CAD build for the part. Positions are in the model's coordinates, mm. A direction names the side the tool comes from. Round coordinates to 2 decimals unless told otherwise and drop trailing zeros. Order: outer loops, then holes, each group sorted by start corner. A loop starts at its lowest first (then second) coordinate and runs counter-clockwise, first axis right, second up. Notation, with made-up numbers: (-3, 66.25) -> (33, 66.25) arc R22 ccw to (33, 103.25) -> close; hole circle Ø4 at (-12.5, -4.75). An arc over 180 degrees is marked (long way). Return JSON: item names as keys, results as strings. Group by question number.
Q1. Flat gauge pins, fed straight in: pin 1 (1.2 mm diameter, centred on x = 84.5, z = 1.5, fed in from -Y); pin 2 (5 mm diameter, centred on x = 53.5, y = 19.25, fed in from +Z); pin 3 (2.5 mm diameter, centred on x = 4.5, y = 19.25, fed in from -Z). Where does each tip first touch, or does it go through?
Q2. Which spindle directions (+Z, -Z, +X, -X, +Y, -Y) get a long thin tool onto all of the face, cutting with end or side? Do faces 1 (the flat face through (29, 0, 2)), 2 (the flat face through (8.5, 8, 2)). Say none if no direction does.
Q3. Cut at C-C (y = 8.75). Write the cut outline in (x, z), then the cut area to 3 significant figures.
Q4. Cut at B-B (x = 158.5). Write the cut outline in (y, z), then the cut area to 3 significant figures.
Q5. Probe line 1 along X through (y, z) = (6.5, 3); line 2 along Y through (x, z) = (175.5, 1.7); line 3 along Y through (x, z) = (126.5, 1.3). List the from-to ranges inside material, lowest first.
Q6. Mould opens along Y. For faces 3 (the flat face through (90, 4, 2)), 4 (the flat face through (29, 3.75, 2)), 5 (the flat face through (90, 24, 2)) say: +Y half, -Y half, draft (parallel to the pull), parting line (faces both ways), or undercut.
Q7. Cut at D-D (z = 3). Count the separate pieces of the cut face and the enclosed holes in it, then the cut area to 3 significant figures.
Q8. Cut at A-A (y = 22.5). Write the cut outline in (x, z), then the cut area to 3 significant figures.
from build123d import *

# Parameters (mm, degrees)
SKETCH1_R           = 1.5
BOSS_EXTRUDE1_DEPTH = 4


with BuildPart() as part:
    # Sketch1 → Boss-Extrude1 (new body)
    with BuildSketch(Plane.XY):
        with BuildLine():
            Line((0, 2), (0, 26))
            ThreePointArc((0, 26), (0.585786438, 27.414213562), (2, 28))
            Line((2, 28), (56, 28))
            ThreePointArc((56, 28), (57.414213562, 27.414213562), (58, 26))
            ThreePointArc((58, 26), (58.585786438, 24.585786438), (60, 24))
            Line((60, 24), (120, 24))
            ThreePointArc((120, 24), (121.414213562, 24.585786438), (122, 26))
            ThreePointArc((122, 26), (122.585786438, 27.414213562), (124, 28))
            Line((124, 28), (178, 28))
            ThreePointArc((178, 28), (179.414213562, 27.414213562), (180, 26))
            Line((180, 26), (180, 2))
            ThreePointArc((180, 2), (179.414213562, 0.585786438), (178, 0))
            Line((178, 0), (124, 0))
            ThreePointArc((124, 0), (122.585786438, 0.585786438), (122, 2))
            ThreePointArc((122, 2), (121.414213562, 3.414213562), (120, 4))
            Line((120, 4), (60, 4))
            ThreePointArc((60, 4), (58.585786438, 3.414213562), (58, 2))
            ThreePointArc((58, 2), (57.414213562, 0.585786438), (56, 0))
            Line((56, 0), (2, 0))
            ThreePointArc((2, 0), (0.585786438, 0.585786438), (0, 2))
        make_face()
        with Locations((53.5, 19.25)):
            Circle(SKETCH1_R, mode=Mode.SUBTRACT)
        with Locations((53.5, 8.75)):
            Circle(SKETCH1_R, mode=Mode.SUBTRACT)
        with Locations((4.5, 19.25)):
            Circle(SKETCH1_R, mode=Mode.SUBTRACT)
        with Locations((4.5, 8.75)):
            Circle(SKETCH1_R, mode=Mode.SUBTRACT)
        with Locations((175.5, 19.25)):
            Circle(SKETCH1_R, mode=Mode.SUBTRACT)
        with Locations((175.5, 8.75)):
            Circle(SKETCH1_R, mode=Mode.SUBTRACT)
        with Locations((126.5, 19.25)):
            Circle(SKETCH1_R, mode=Mode.SUBTRACT)
        with Locations((126.5, 8.75)):
            Circle(SKETCH1_R, mode=Mode.SUBTRACT)
        with Locations((60, 14)):
            Circle(SKETCH1_R, mode=Mode.SUBTRACT)
        with Locations((120, 14)):
            Circle(SKETCH1_R, mode=Mode.SUBTRACT)
        with Locations((175.5, 3.75)):
            Circle(SKETCH1_R, mode=Mode.SUBTRACT)
        Polygon((8.5, 3.75), (8.5, 12.75), (5, 12.75), (5, 15.25), (8.5, 15.25), (8.5, 24.25), (49.5, 24.25), (49.5, 15.25), (53, 15.25), (53, 12.75), (49.5, 12.75), (49.5, 3.75), align=None, mode=Mode.SUBTRACT)
        Polygon((130.5, 3.75), (130.5, 12.75), (127, 12.75), (127, 15.25), (130.5, 15.25), (130.5, 24.25), (171.5, 24.25), (171.5, 15.25), (175, 15.25), (175, 12.75), (171.5, 12.75), (171.5, 3.75), align=None, mode=Mode.SUBTRACT)
    extrude(amount=BOSS_EXTRUDE1_DEPTH)


solid = part.part
Solution:
{
 "1": {"pin 1": "stops at y = 4", "pin 2": "stops at z = 4", "pin 3": "passes through"},
 "2": {"face 1": "+Z, -Z, +X, -X, -Y", "face 2": "+Z, -Z"},
 "3": {"outline": "(0, 0) -> (3, 0) -> (3, 4) -> (0, 4) -> close; (6, 0) -> (8.5, 0) -> (8.5, 4) -> (6, 4) -> close; (49.5, 0) -> (52, 0) -> (52, 4) -> (49.5, 4) -> close; (55, 0) -> (125, 0) -> (125, 4) -> (55, 4) -> close; (128, 0) -> (130.5, 0) -> (130.5, 4) -> (128, 4) -> close; (171.5, 0) -> (174, 0) -> (174, 4) -> (171.5, 4) -> close; (177, 0) -> (180, 0) -> (180, 4) -> (177, 4) -> close", "area": "344 mm²"},
 "4": {"outline": "(0, 0) -> (3.75, 0) -> (3.75, 4) -> (0, 4) -> close; (24.25, 0) -> (28, 0) -> (28, 4) -> (24.25, 4) -> close", "area": "30.0 mm²"},
 "5": {"line 1": "x = 0 to 8.5, 49.5 to 130.5, 171.5 to 180", "line 2": "y = 0 to 2.25, 5.25 to 7.25, 10.25 to 17.75, 20.75 to 28", "line 3": "y = 0 to 7.25, 10.25 to 17.75, 20.75 to 28"},
 "6": {"face 3": "-Y half", "face 4": "undercut", "face 5": "+Y half"},
 "7": {"separate pieces": "1", "enclosed holes": "13", "area": "2,730 mm²"},
 "8": {"outline": "(0, 0) -> (8.5, 0) -> (8.5, 4) -> (0, 4) -> close; (49.5, 0) -> (130.5, 0) -> (130.5, 4) -> (49.5, 4) -> close; (171.5, 0) -> (180, 0) -> (180, 4) -> (171.5, 4) -> close", "area": "392 mm²"}
}
